Could you check a few things on this model? Use its own coordinates, in mm. A direction names the side the tool comes from. Round coordinates to 2 decimals unless told otherwise and drop trailing zeros. Write each loop counter-clockwise with the first axis right and the second up, starting at its lowest first coordinate (ties: lowest second). Pieces come first, ordered by that corner, then holes. Notation, with made-up numbers: (-23, 13) -> (-11, 13) arc R14 ccw to (-11, 21) -> close; hole circle Ø11 at (59, -18.75). An arc over 180 degrees is marked (long way). Answer in a Markdown table with one row per item. Add a question column.
```python
from build123d import *

# Parameters (mm, degrees)
F0_W     = 225
F0_H     = 300
F0_W_2   = 300
F0_H_2   = 450
F1_DEPTH = 665


with BuildPart() as f1:
    # F0 (on Right) → F1 (new body, symmetric)
    with BuildSketch(Plane.YZ):
        with Locations((112.5, 300)):
            Rectangle(F0_W, F0_H)
        Polygon((0, 150), (0, 0), (300, 0), (470, 0), (470, 150), (225, 150), align=None)
        with Locations((150, -225)):
            Rectangle(F0_W_2, F0_H_2)
    extrude(amount=F1_DEPTH, both=True)


solid = f1.part
```
(1) Suppose I cut it at C-C, the plane z = 294.5. Please give me the cut outline in (x, y), then the cut area to 3 significant figures.
(2) Suppose I cut it at B-B, the plane y = 285. Please give me the cut outline in (x, z).
(3) Suppose I cut it at A-A, the plane x = 391.5. Please give me the cut outline in (y, z), then the cut area to 3 significant figures.
(4) For P1, Ø3, axis at x = -60.5, z = -281.5, coming from the +Y side; P2, Ø1.5, axis at x = 439, y = 375, coming from the +Z side, each with a flat end and sliding along its axis, tell me the tip position at first contact or that it passes through.
(5) On a 3-axis mill with a long thin cutter (end or side, diameter ignored), from which of +Z, -Z, +X, -X, +Y, -Y can I reach the whole of each face in a straight line? I mean faces 1 (the face through (9, 148, -450)), 2 (the face through (9, 349, 150)), 3 (the face through (9, 384, 0)). Say none if no direction works.
(6) I need wall thicknesses on L1, parallel to Y at x = -564, z = 230; L2, parallel to Y at x = 318, z = -129; L3, parallel to Z at x = -386, y = 438.5. Which ranges of each line are inside material? Lowest first, please.
Response:
| question | item | result |
|---|---|---|
| 1 | outline | (-665, 0) -> (665, 0) -> (665, 225) -> (-665, 225) -> close |
| 1 | area | 299,000 mm² |
| 2 | outline | (-665, -450) -> (665, -450) -> (665, 150) -> (-665, 150) -> close |
| 3 | outline | (0, -450) -> (300, -450) -> (300, 0) -> (470, 0) -> (470, 150) -> (225, 150) -> (225, 450) -> (0, 450) -> close |
| 3 | area | 273,000 mm² |
| 4 | P1 | y = 300 |
| 4 | P2 | z = 150 |
| 5 | face 1 | -Z, +X, -X, +Y, -Y |
| 5 | face 2 | +Z, +X, -X, +Y |
| 5 | face 3 | -Z, +X, -X, +Y |
| 6 | L1 | 0 to 225 |
| 6 | L2 | 0 to 300 |
| 6 | L3 | 0 to 150 |
